Here's how the part is built. I have some questions about the finished solid (model axes, mm). Round coordinates to 2 decimals unless told otherwise and drop trailing zeros. Write each loop counter-clockwise with the first axis right and the second up, starting at its lowest first coordinate (ties: lowest second). Pieces come first, ordered by that corner, then holes. Notation, with made-up numbers: (-36, 15) -> (16, 15) arc R17 ccw to (16, 42) -> close; hole circle Ø11 at (2.5, 21). An arc over 180 degrees is marked (long way). Answer as CSV lines item,"result".
from build123d import *

# Parameters (mm, degrees)
ESQUISSE1_R        = 1.55
BOSS_EXTRU_1_DEPTH = 3


with BuildPart() as part:
    # Esquisse1 → Boss.-Extru.1 (new body)
    with BuildSketch(Plane.XY):
        with BuildLine():
            Line((-46.5, 25.5), (-46.5, -25.5))
            ThreePointArc((-46.5, -25.5), (-45.914213562, -26.914213562), (-44.5, -27.5))
            Line((-44.5, -27.5), (44.5, -27.5))
            ThreePointArc((44.5, -27.5), (45.914213562, -26.914213562), (46.5, -25.5))
            Line((46.5, -25.5), (46.5, 25.5))
            ThreePointArc((46.5, 25.5), (45.914213562, 26.914213562), (44.5, 27.5))
            Line((44.5, 27.5), (-44.5, 27.5))
            ThreePointArc((-44.5, 27.5), (-45.914213562, 26.914213562), (-46.5, 25.5))
        make_face()
        with Locations((-42.5, 23.5)):
            Circle(ESQUISSE1_R, mode=Mode.SUBTRACT)
        with Locations((-42.5, -23.5)):
            Circle(ESQUISSE1_R, mode=Mode.SUBTRACT)
        with Locations((42.5, 23.5)):
            Circle(ESQUISSE1_R, mode=Mode.SUBTRACT)
        with Locations((42.5, -23.5)):
            Circle(ESQUISSE1_R, mode=Mode.SUBTRACT)
        with BuildLine():
            Line((31, 19.5), (2, 19.5))
            ThreePointArc((2, 19.5), (0.585786438, 18.914213562), (0, 17.5))
            Line((0, 17.5), (0, 3.5))
            ThreePointArc((0, 3.5), (0.585786438, 2.085786438), (2, 1.5))
            Line((2, 1.5), (22.413214262, 1.5))
            ThreePointArc((22.413214262, 1.5), (23.827427824, 0.914213562), (24.413214262, -0.5))
            Line((24.413214262, -0.5), (24.413214262, -20.5))
            ThreePointArc((24.413214262, -20.5), (24.999000699, -21.914213562), (26.413214262, -22.5))
            Line((26.413214262, -22.5), (31, -22.5))
            ThreePointArc((31, -22.5), (32.414213562, -21.914213562), (33, -20.5))
            Line((33, -20.5), (33, 17.5))
            ThreePointArc((33, 17.5), (32.414213562, 18.914213562), (31, 19.5))
        make_face(mode=Mode.SUBTRACT)
    extrude(amount=BOSS_EXTRU_1_DEPTH)


solid = part.part
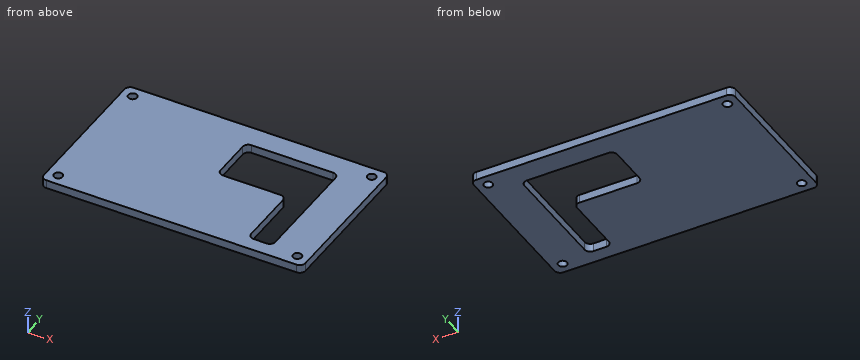
Item 1: Suppose I cut it at C-C, the plane x = -42.5. List the corners of the cut face in (y, z) for me, then the cut area to 3 significant figures.
Results found:
outline,"(-27.5, 0) -> (-25.05, 0) -> (-25.05, 3) -> (-27.5, 3) -> close; (-21.95, 0) -> (21.95, 0) -> (21.95, 3) -> (-21.95, 3) -> close; (25.05, 0) -> (27.5, 0) -> (27.5, 3) -> (25.05, 3) -> close"
area,"146 mm²"
Item 2: Suppose I cut it at D-D, the plane z = 0.7. List the corners of the cut face in (x, y) for me.
Results found:
outline,"(-46.5, -25.5) arc R2 ccw to (-44.5, -27.5) -> (44.5, -27.5) arc R2 ccw to (46.5, -25.5) -> (46.5, 25.5) arc R2 ccw to (44.5, 27.5) -> (-44.5, 27.5) arc R2 ccw to (-46.5, 25.5) -> close; hole circle Ø3.1 at (-42.5, -23.5); hole circle Ø3.1 at (-42.5, 23.5); hole (0, 3.5) arc R2 ccw to (2, 1.5) -> (22.41, 1.5) arc R2 cw to (24.41, -0.5) -> (24.41, -20.5) arc R2 ccw to (26.41, -22.5) -> (31, -22.5) arc R2 ccw to (33, -20.5) -> (33, 17.5) arc R2 ccw to (31, 19.5) -> (2, 19.5) arc R2 ccw to (0, 17.5) -> close; hole circle Ø3.1 at (42.5, -23.5); hole circle Ø3.1 at (42.5, 23.5)"
Item 3: Suppose I cut it at A-A, the plane x = 18.5. List the corners of the cut face in (y, z) for me.
Results found:
outline,"(-27.5, 0) -> (1.5, 0) -> (1.5, 3) -> (-27.5, 3) -> close; (19.5, 0) -> (27.5, 0) -> (27.5, 3) -> (19.5, 3) -> close"
Item 4: Suppose I cut it at B-B, the plane y = 12. List the corners of the cut face in (x, z) for me, then the cut area to 3 significant figures.
Results found:
outline,"(-46.5, 0) -> (0, 0) -> (0, 3) -> (-46.5, 3) -> close; (33, 0) -> (46.5, 0) -> (46.5, 3) -> (33, 3) -> close"
area,"180 mm²"
Item 5: I need wall thicknesses on L1, parallel to Y at x = -42.5, z = 0.95; L2, parallel to X at y = -14, z = 2.3; L3, parallel to X at y = 7, z = 1.95. Which ranges of each line are inside material? Lowest first, please.
Results found:
L1,"y = -27.5 to -25.05, -21.95 to 21.95, 25.05 to 27.5"
L2,"x = -46.5 to 24.41, 33 to 46.5"
L3,"x = -46.5 to 0, 33 to 46.5"
Item 6: Will these pins go through, and if not, where does the flat tip stop? pin 1 (2.5 mm diameter, centred on x = -42.5, y = 23.5, fed in from +Z); pin 2 (5 mm diameter, centred on x = 42.5, y = 23.5, fed in from -Z).
Results found:
pin 1,"passes through"
pin 2,"stops at z = 0"
